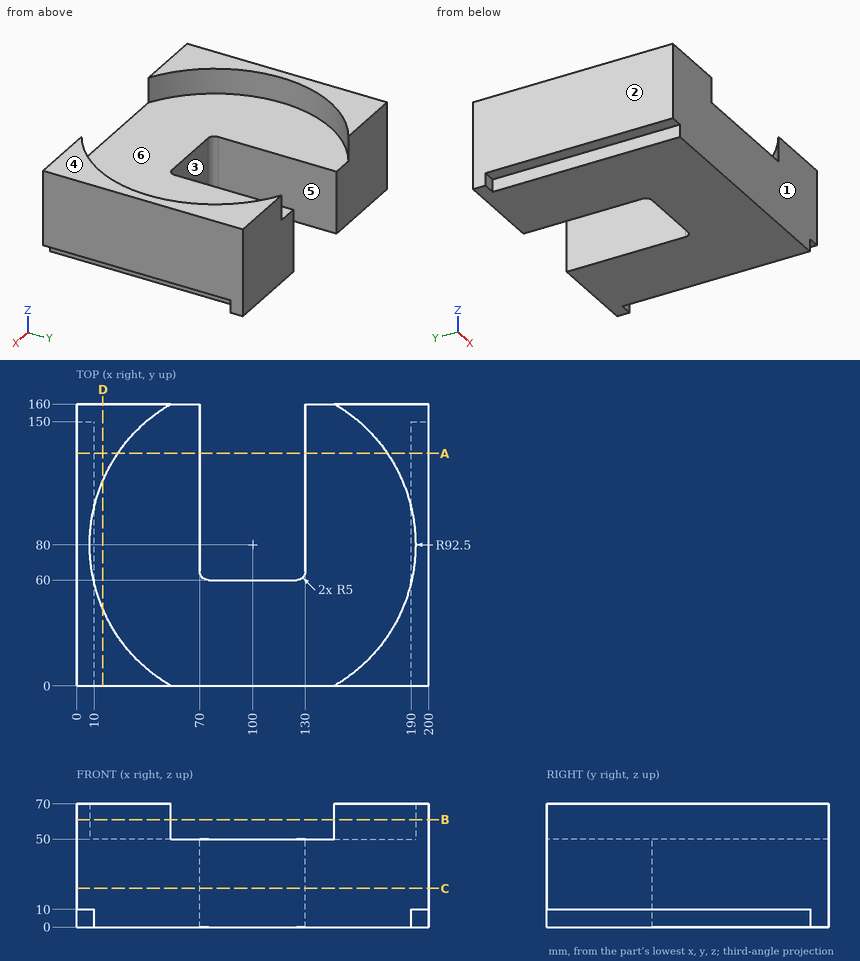
Drawing for the job (mm, zero at the part's lowest x, y, z). A direction names the side the tool comes from. Give positions to 0.01 mm unless a question says otherwise; leave off trailing zeros. Loops run counter-clockwise (first coordinate to the right, second up) from the corner with the lowest first, then second, coordinate; pieces in that order, holes last.
(1) Band-saw the part on B-B (z = 61). Write the cut outline in (x, y), and give its area (3 significant figures).
Return value:
outline: (0, 0) - (53.56, 0) arc R92.5 cw to (53.56, 160) - (0, 160) - close; (146.44, 0) - (200, 0) - (200, 160) - (146.44, 160) arc R92.5 cw to start
area: 6,690 mm2
(2) Band-saw the part on A-A (y = 132). Write the cut outline in (x, z), and give its area (3 significant figures).
Return value:
outline: (0, 10) - (10, 10) - (10, 0) - (70, 0) - (70, 50) - (23.5, 50) - (23.5, 70) - (0, 70) - close; (130, 0) - (190, 0) - (190, 10) - (200, 10) - (200, 70) - (176.5, 70) - (176.5, 50) - (130, 50) - close
area: 7,740 mm2
(3) 3-axis set-ups, long thin cutter, end or side, ignore diameter. For the marked faces 4, 5 and 6: which of +Z, -Z, +X, -X, +Y, -Y reach the whole face in a straight line?
Return value:
face 4: +Z, +X, -X, +Y, -Y
face 5: +Z, -Z, +Y
face 6: +Z
(4) Band-saw the part on C-C (z = 22). Write the cut outline in (x, y).
Return value:
outline: (0, 0) - (200, 0) - (200, 160) - (130, 160) - (130, 65) arc R5 cw to (125, 60) - (75, 60) arc R5 cw to (70, 65) - (70, 160) - (0, 160) - close
(5) Pull direction X, two halves, no side cores. Call the marked faces 1, 2 and 3: pulls with the +X half, pulls with the -X half, needs draft (parallel to the pull), parting line crosses it, or undercut.
Return value:
face 1: needs draft
face 2: pulls with the -X half
face 3: undercut
(6) Band-saw the part on D-D (x = 15). Write the cut outline in (y, z), and give its area (3 significant figures).
Return value:
outline: (0, 0) - (160, 0) - (160, 70) - (116.49, 70) - (116.49, 50) - (43.51, 50) - (43.51, 70) - (0, 70) - close
area: 9,740 mm2
(7) Pin check, flat tips, straight feed: pin 1 (3 mm diameter, centred on y = 44.5, z = 6.5, fed in from +X); pin 2 (5 mm diameter, centred on x = 196, z = 5.5, fed in from -Y); pin 3 (5 mm diameter, centred on x = 68.5, y = 56, fed in from +Z). Stop position of each tip, or through.
Return value:
pin 1: stops at x = 190
pin 2: stops at y = 150
pin 3: stops at z = 50
(8) Drill centre lines: line 1 along X through (y, z) = (120, 26.5); line 2 along Z through (x, y) = (16, 90); line 3 along Y through (x, z) = (92.5, 44). Where is each one in solid material? Low to high.
Return value:
line 1: x = 0 to 70, 130 to 200
line 2: z = 0 to 50
line 3: y = 0 to 60
